The model under review builds one solid part; all positions refer to its coordinate system, in mm. Face numbers are marked on the shaded views. A direction names the side the tool comes from. Give positions to 0.01 mm unless a question says otherwise; leave off trailing zeros. Loops run counter-clockwise (first coordinate to the right, second up) from the corner with the lowest first, then second, coordinate; pieces in that order, holes last. Notation, with made-up numbers: (25.5, 81.5) -> (64.5, 81.5) arc R4 ccw to (64.5, 86.5) -> close; hole circle Ø9 at (-11, 45.25). An arc over 180 degrees is marked (long way). Write each question's results on one line, items separated by ' | '. Start each with the question number.
Q1. We need section B-B (x = 6). Write out the cut boundary in (y, z), plus the area to 4 significant figures.
Q2. Insertion check: pin 1 Ø1.6 at (x, z) = (49.5, -0.5) entering from -Y; pin 2 Ø6.5 at (x, z) = (5.5, -63.5) entering from +Y; pin 3 Ø10 at (x, z) = (24.5, -69.5) entering from +Y. Each pin has a flat end and moves straight along its axis. Give the tip position at first contact, or say it passes through.
Q3. We need section A-A (z = -6). Write out the cut boundary in (x, y).
Q4. We need section C-C (x = 64). Write out the cut boundary in (y, z).
Q5. Machinability: for the marked faces 5 and 6, which of the approach directions +Z, -Z, +X, -X, +Y, -Y give a long, thin tool a straight path to every point of the face, cutting with its end or side? Answer none if there is none.
Q6. Mouldability with a two-part tool opening along X and no side actions: class the marked faces 1, 2, 3 and 4 as released by +X, released by -X, zero draft, split by the parting line, or undercut.
Q7. Wall thickness on L1, parallel to Z at x = 6.5, y = 11.5; L2, parallel to Z at x = 94, y = -0.7; L3, parallel to X at y = 15.5, z = -13: over which ranges is each line inside the solid? List them lowest first. Write a range as [from, to].
Q8. We need section D-D (z = -46). Write out the cut boundary in (x, y), plus the area to 3 significant figures.
from build123d import *

# Parameters (mm, degrees)
ESQUISSE1_W             = 100
ESQUISSE1_H             = 80
ESQUISSE1_R             = 1.75
ESQUISSE1_R_2           = 1.25
ESQUISSE1_W_2           = 15
ESQUISSE1_H_2           = 10
BOSS_EXTRU_1_DEPTH      = 1.5
BOSS_EXTRU_2_DEPTH      = 36.5
ESQUISSE3_R             = 1.25
ESQUISSE3_W             = 32
ESQUISSE3_H             = 12
ENL_V_MAT_EXTRU_1_DEPTH = 5
ESQUISSE4_W             = 96
ESQUISSE4_H             = 76
ESQUISSE4_R             = 1.75
ESQUISSE4_R_2           = 1.25
ESQUISSE4_W_2           = 15
ESQUISSE4_H_2           = 10
BOSS_EXTRU_3_DEPTH      = 1.5
ENL_V_MAT_EXTRU_2_DEPTH = 1.5
ESQUISSE6_W             = 5
ESQUISSE6_H             = 4.5
ENL_V_MAT_EXTRU_3_DEPTH = 10


with BuildPart() as part:
    # Esquisse1 → Boss.-Extru.1 (new body)
    with BuildSketch(Plane(origin=(0, 0, 0), x_dir=(1, 0, 0), z_dir=(0, 1, 0))):
        with Locations((50, 40)):
            Rectangle(ESQUISSE1_W, ESQUISSE1_H)
        with Locations((6, 74)):
            Circle(ESQUISSE1_R, mode=Mode.SUBTRACT)
        with Locations((94, 74)):
            Circle(ESQUISSE1_R, mode=Mode.SUBTRACT)
        with Locations((94, 6)):
            Circle(ESQUISSE1_R, mode=Mode.SUBTRACT)
        with Locations((6, 6)):
            Circle(ESQUISSE1_R, mode=Mode.SUBTRACT)
        with Locations((88, 26.081709878)):
            Circle(ESQUISSE1_R, mode=Mode.SUBTRACT)
        with Locations((39, 26.081709878)):
            Circle(ESQUISSE1_R, mode=Mode.SUBTRACT)
        with Locations((39, 49.081709878)):
            Circle(ESQUISSE1_R, mode=Mode.SUBTRACT)
        with Locations((28.72, 37.850032574)):
            Circle(ESQUISSE1_R_2, mode=Mode.SUBTRACT)
        with Locations((12, 52.360032574)):
            Circle(ESQUISSE1_R_2, mode=Mode.SUBTRACT)
        with Locations((50, 70)):
            Rectangle(ESQUISSE1_W_2, ESQUISSE1_H_2, mode=Mode.SUBTRACT)
    extrude(amount=BOSS_EXTRU_1_DEPTH)

    # Esquisse2 → Boss.-Extru.2 (add)
    with BuildSketch(Plane(origin=(0, 1.5, 0), x_dir=(1, 0, 0), z_dir=(0, 1, 0))):
        Polygon((1.5, 78.5), (98.5, 78.5), (98.5, 67.5), (92.5, 67.5), (92.5, 64.5), (92.5, 61.5), (95.5, 61.5), (95.5, 64.5), (98.5, 64.5), (98.5, 61.5), (100, 61.5), (100, 80), (0, 80), (0, 61.5), (1.5, 61.5), (1.5, 64.5), (4.5, 64.5), (4.5, 61.5), (7.5, 61.5), (7.5, 64.5), (7.5, 67.5), (1.5, 67.5), align=None)
        Polygon((1.5, 1.5), (98.5, 1.5), (98.5, 13.5), (92.5, 13.5), (92.5, 16.5), (92.5, 19.237081293), (95.5, 19.237081293), (95.5, 16.5), (98.5, 16.5), (98.5, 19.237081293), (100, 19.237081293), (100, 0), (0, 0), (0, 19.5), (1.5, 19.5), (1.5, 16.5), (4.5, 16.5), (4.5, 19.5), (7.5, 19.5), (7.5, 16.5), (7.5, 13.5), (1.5, 13.5), align=None)
    extrude(amount=BOSS_EXTRU_2_DEPTH)

    # Esquisse3 → Enlèv. mat.-Extru.1 (cut)
    with BuildSketch(Plane.XY):
        with Locations((34, 29)):
            Circle(ESQUISSE3_R)
        with Locations((34, 12)):
            Circle(ESQUISSE3_R)
        with Locations((64, 12)):
            Circle(ESQUISSE3_R)
        with Locations((64, 29)):
            Circle(ESQUISSE3_R)
        with Locations((50, 21)):
            Rectangle(ESQUISSE3_W, ESQUISSE3_H)
    extrude(amount=-ENL_V_MAT_EXTRU_1_DEPTH, mode=Mode.SUBTRACT)

    # Esquisse4 → Boss.-Extru.3 (add)
    with BuildSketch(Plane.XZ):
        with Locations((50, -40)):
            Rectangle(ESQUISSE4_W, ESQUISSE4_H)
        with Locations((6, -6)):
            Circle(ESQUISSE4_R, mode=Mode.SUBTRACT)
        with Locations((6, -74)):
            Circle(ESQUISSE4_R, mode=Mode.SUBTRACT)
        with Locations((94, -74)):
            Circle(ESQUISSE4_R, mode=Mode.SUBTRACT)
        with Locations((94, -6)):
            Circle(ESQUISSE4_R, mode=Mode.SUBTRACT)
        with Locations((88, -26.081709878)):
            Circle(ESQUISSE4_R, mode=Mode.SUBTRACT)
        with Locations((39, -49.081709878)):
            Circle(ESQUISSE4_R, mode=Mode.SUBTRACT)
        with Locations((39, -26.081709878)):
            Circle(ESQUISSE4_R, mode=Mode.SUBTRACT)
        with Locations((28.72, -37.850032574)):
            Circle(ESQUISSE4_R_2, mode=Mode.SUBTRACT)
        with Locations((12, -52.360032574)):
            Circle(ESQUISSE4_R_2, mode=Mode.SUBTRACT)
        with Locations((50, -70)):
            Rectangle(ESQUISSE4_W_2, ESQUISSE4_H_2, mode=Mode.SUBTRACT)
    extrude(amount=BOSS_EXTRU_3_DEPTH)

    # Esquisse5 → Enlèv. mat.-Extru.2 (cut)
    with BuildSketch(Plane(origin=(0, 38, 0), x_dir=(1, 0, 0), z_dir=(0, 1, 0))):
        Polygon((1.5, 67.5), (7.5, 67.5), (7.5, 64.5), (7.5, 61.5), (4.5, 61.5), (4.5, 64.5), (1.5, 64.5), align=None)
        Polygon((1.5, 16.5), (4.5, 16.5), (4.5, 19.5), (7.5, 19.5), (7.5, 16.503082132), (7.5, 13.5), (1.5, 13.5), align=None)
        Polygon((92.5, 19.237081293), (95.5, 19.237081293), (95.5, 16.5), (98.5, 16.5), (98.5, 13.5), (92.5, 13.5), align=None)
        Polygon((95.5, 61.5), (92.5, 61.5), (92.5, 67.5), (95.5, 67.5), (98.5, 67.5), (98.5, 64.5), (95.5, 64.5), align=None)
    extrude(amount=-ENL_V_MAT_EXTRU_2_DEPTH, mode=Mode.SUBTRACT)

    # Esquisse6 → Enlèv. mat.-Extru.3 (cut)
    with BuildSketch(Plane.XY.offset(-78.5)):
        with Locations((35.5, 35.75)):
            Rectangle(ESQUISSE6_W, ESQUISSE6_H)
        with Locations((64.5, 35.75)):
            Rectangle(ESQUISSE6_W, ESQUISSE6_H)
    extrude(amount=-ENL_V_MAT_EXTRU_3_DEPTH, mode=Mode.SUBTRACT)


solid = part.part
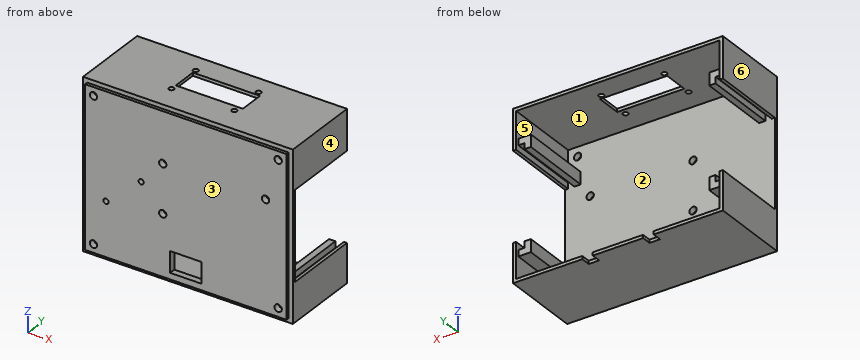
Output:
1) outline: (-1.5, -78) -> (0, -78) -> (0, -80) -> (38, -80) -> (38, -78.5) -> (1.5, -78.5) -> (1.5, -75.75) -> (-1.5, -75.75) -> close; (-1.5, -72.25) -> (1.5, -72.25) -> (1.5, -67.5) -> (36.5, -67.5) -> (36.5, -61.5) -> (1.5, -61.5) -> (1.5, -19.5) -> (36.5, -19.5) -> (36.5, -13.5) -> (1.5, -13.5) -> (1.5, -7.75) -> (-1.5, -7.75) -> close; (-1.5, -4.25) -> (1.5, -4.25) -> (1.5, -1.5) -> (38, -1.5) -> (38, 0) -> (0, 0) -> (0, -2) -> (-1.5, -2) -> close | area: 742.5 mm2
2) pin 1: y = 0 | pin 2: y = 36.5 | pin 3: y = 1.5
3) outline: (0, 0) -> (2, 0) -> (2, -1.5) -> (4.25, -1.5) -> (4.25, 1.5) -> (1.5, 1.5) -> (1.5, 38) -> (0, 38) -> close; (7.75, -1.5) -> (92.25, -1.5) -> (92.25, 1.5) -> (7.75, 1.5) -> close; (95.75, -1.5) -> (98, -1.5) -> (98, 0) -> (100, 0) -> (100, 38) -> (98.5, 38) -> (98.5, 1.5) -> (95.75, 1.5) -> close
4) outline: (-1.5, -78) -> (0, -78) -> (0, -80) -> (33.5, -80) -> (33.5, -78.5) -> (1.5, -78.5) -> (1.5, -1.5) -> (10.75, -1.5) -> (10.75, 0) -> (0, 0) -> (0, -2) -> (-1.5, -2) -> close; (13.25, -1.5) -> (15, -1.5) -> (15, 0) -> (13.25, 0) -> close; (27, -1.5) -> (27.75, -1.5) -> (27.75, 0) -> (27, 0) -> close; (30.25, -1.5) -> (38, -1.5) -> (38, 0) -> (30.25, 0) -> close
5) face 5: +Y | face 6: +Z, -Z, -X, +Y, -Y
6) face 1: undercut | face 2: undercut | face 3: zero draft | face 4: released by +X
7) L1: [-80, -78.5], [-67.5, -61.5], [-19.5, -13.5], [-1.5, 0] | L2: [-78, -75.75], [-72.25, -7.75], [-4.25, -2] | L3: [0, 1.5], [98.5, 100]
8) outline: (0, 0) -> (2, 0) -> (2, -1.5) -> (98, -1.5) -> (98, 0) -> (100, 0) -> (100, 1.5) -> (0, 1.5) -> close | area: 294 mm2
